Check sheet for the modelled part. Datum: model origin and axes. Units: mm. Give positions to 0.01 mm unless a question says otherwise; leave off trailing zeros. Write each loop counter-clockwise with the first axis right and the second up, starting at its lowest first coordinate (ties: lowest second). Pieces come first, ordered by that corner, then holes. Notation, with made-up numbers: M 9.5,26.5 L 61.5,26.5 A24 ccw 61.5,52.5 Z; hole C 51.5,56.5 d9. An arc over 180 degrees is marked long. Write item = value, one per line. Start each with the question number.
1) Go/stop test with flat-tipped pins: pin 1 (3 mm diameter, centred on x = 0, y = 0, fed in from +Z); pin 2 (2 mm diameter, centred on y = -1.5, z = 1.5, fed in from +X); pin 3 (1 mm diameter, centred on y = -6, z = 2, fed in from +X). Record where each tip stops, or that it passes through.
2) Cross-section at C-C, the plane y = -5.75. Record the cut outline in (x, z), plus the area to 3 significant figures.
3) Cross-section at A-A, the plane x = 0. Record the cut outline in (y, z).
4) Cross-section at B-B, the plane z = 2.25. Record the cut outline in (x, y).
5) Mould release check, pull along X, two halves, no side actions. Record for faces 1 (the cylindrical face through (5, 0, 2)), 2 (the flat face through (-15, 13, 2)), 3 (the cylindrical face through (0, -5, 2)), 4 (the flat face through (-13, -15, 2)): released by +X, released by -X, zero draft, split by the parting line, or undercut.
6) Scan lines: line 1 along Y through (x, z) = (0, 3); line 2 along Y through (x, z) = (-10.25, 1.6); line 3 along X through (y, z) = (13, 1.95). Record each from-to range of solid material in increasing order. Write a range as [from, to].
```python
from build123d import *

# Parameters (mm, degrees)
F0_R     = 2.5
F1_DEPTH = 4


with BuildPart() as f1:
    # F0 (on Top) → F1 (new body)
    with BuildSketch(Plane.XY):
        with BuildLine():
            Line((15, 10), (15, 15))
            Line((15, 15), (10, 15))
            ThreePointArc((10, 15), (0, 5), (-10, 15))
            Line((-10, 15), (-15, 15))
            Line((-15, 15), (-15, 10))
            ThreePointArc((-15, 10), (-7.928932, 7.071068), (-5, 0))
            ThreePointArc((-5, 0), (-7.928932, -7.071068), (-15, -10))
            Line((-15, -10), (-15, -15))
            Line((-15, -15), (-10, -15))
            ThreePointArc((-10, -15), (0, -5), (10, -15))
            Line((10, -15), (15, -15))
            Line((15, -15), (15, -10))
            ThreePointArc((15, -10), (5, 0), (15, 10))
        make_face()
        Circle(F0_R, mode=Mode.SUBTRACT)
    extrude(amount=F1_DEPTH)


solid = f1.part
```
Reply:
q1.pin_1 = through
q1.pin_2 = 5.32
q1.pin_3 = 7.4
q2.outline = M -6.82,0 L -3.8,0 L -3.8,4 L -6.82,4 Z; M 3.8,0 L 6.82,0 L 6.82,4 L 3.8,4 Z
q2.area = 24.2 mm2
q3.outline = M -5,0 L -2.5,0 L -2.5,4 L -5,4 Z; M 2.5,0 L 5,0 L 5,4 L 2.5,4 Z
q4.outline = M -15,-15 L -10,-15 A10 cw 10,-15 L 15,-15 L 15,-10 A10 cw 15,10 L 15,15 L 10,15 A10 cw -10,15 L -15,15 L -15,10 A10 cw -5,0 A10 cw -15,-10 Z; hole C 0,0 d5
q5.face_1 = released by +X
q5.face_2 = released by -X
q5.face_3 = undercut
q5.face_4 = zero draft
q6.line_1 = [-5, -2.5], [2.5, 5]
q6.line_2 = [-15, -8.8], [8.8, 15]
q6.line_3 = [-15, -9.8], [9.8, 15]
